Part model, mm, in its own coordinate system. Face numbers are marked on the shaded views. A direction names the side the tool comes from. Coordinates: 2 decimals unless noted, no trailing zeros. Order: outer loops, then holes, each group sorted by start corner. A loop starts at its lowest first (then second) coordinate and runs counter-clockwise, first axis right, second up. Notation, with made-up numbers: (0, 55.25) - (43, 55.25) arc R30 cw to (43, 83.25) - close; hole circle Ø1 at (18.5, 1.5). An arc over 180 degrees is marked (long way). Use a Markdown table: item, result. Add a question column.
1) Saw through at A-A on y = 11. List the corners of the cut face in (x, z), then the cut area to 3 significant figures.
2) Saw through at B-B on x = 15. List the corners of the cut face in (y, z), then the cut area to 3 significant figures.
3) Tool access for the marked faces 5, 6 and 7: list every direction of +Z, -Z, +X, -X, +Y, -Y with a clear straight run to the whole face (end or side of a thin tool).
4) Saw through at C-C on z = 17.5. List the corners of the cut face in (x, y), then the cut area to 3 significant figures.
5) Drop flat-ended pins along their axis: P1, Ø6, axis at x = 21, z = -7, coming from the +Y side; P2, Ø3.5, axis at x = 36.5, y = 15.5, coming from the +Z side; P3, Ø1.6, axis at y = 26, z = 26.5, coming from the +X side. Give the stop position or say it passes through.
6) Two-plate mould, pull along X, no slides. Class the marked faces 1, 2, 3 and 4: +X half, -X half, draft (parallel to the pull), parting line (faces both ways), or undercut.
7) Wall check: L1, parallel to X at y = 11.5, z = -5; L2, parallel to Z at x = -40, y = 21.5; L3, parallel to Z at x = -40, y = 25.5. Give the ranges that are in metal, low to high. Write a range as [from, to].
Autodesk Inventor part; units mm, degrees
ref_plane "YZ Plane" through (0, 0, 0) normal (1, 0, 0) x (0, 1, 0)
ref_plane "XZ Plane" through (0, 0, 0) normal (0, 1, 0) x (-1, 0, 0)
ref_plane "XY Plane" through (0, 0, 0) normal (0, 0, 1) x (1, 0, 0)
sketch "Sketch1" plane through (0, 0, 0) normal (0, 1, 0) x (-1, 0, 0)
  line L0 (42.5, 21.5) -> (-42.5, 21.5)
  line L1 (-42.5, 21.5) -> (-42.5, -21.5)
  line L2 (-42.5, -21.5) -> (42.5, -21.5)
  line L3 (42.5, -21.5) -> (42.5, 21.5)
  point P0 (0, 0)
  point P1 (0, -21.5)
  point P2 (42.5, 0)
  dimension "d0" = 43
  dimension "d1" = 85
extrude "Extrusion1" add sketch "Sketch1" along normal blind 4
sketch "Sketch2" plane through (-42.5, 0, 21.5) normal (0, 0, 1) x (1, 0, 0)
  line L0 (0, 25) -> (85, 25)
  line L1 (85, 25) -> (85, 0)
  line L2 (85, 0) -> (0, 0)
  line L3 (0, 0) -> (0, 25)
  point P0 (42.5, 0)
  dimension "d4" = 25
extrude "Extrusion2" add sketch "Sketch2" along normal blind 2
sketch "Sketch3" plane through (42.5, 0, -21.5) normal (0, 0, -1) x (-1, 0, 0)
  line L0 (0, 25) -> (85, 25)
  line L1 (0, 0) -> (85, 0)
  line L2 (0, 25) -> (85, 25)
  line L3 (85, 25) -> (85, 0)
  line L4 (85, 0) -> (0, 0)
  line L5 (0, 0) -> (0, 25)
  point P0 (42.5, 0)
extrude "Extrusion3" add sketch "Sketch3" along normal blind 2
sketch "Sketch4" plane through (-42.5, 25, -21.5) normal (0, 1, 0) x (1, 0, 0)
  line L0 (0, -45) -> (0, 2)
  line L1 (0, 7.62) -> (85, 7.62)
  line L2 (85, 7.62) -> (85, 0)
  line L3 (85, 0) -> (0, 0)
  line L4 (0, 0) -> (0, 7.62)
  point P0 (42.5, -21.5)
  point P1 (85, 3.81)
  point P2 (85, 2)
  dimension "d15" = 7.62
extrude "Extrusion4" add sketch "Sketch4" along normal blind 2
sketch "Sketch5" plane through (-42.5, 25, 21.5) normal (0, 1, 0) x (1, 0, 0)
  line L0 (0, -2) -> (0, 45)
  line L1 (0, 0) -> (85, 0)
  line L2 (85, 0) -> (85, -7.62)
  line L3 (85, -7.62) -> (0, -7.62)
  line L4 (0, -7.62) -> (0, 0)
  line L5 (85, 0) -> (85, -2)
  line L6 (85, 0) -> (0, 0)
  point P0 (42.5, 21.5)
  point P1 (85, -3.81)
  point P2 (85, -1)
  point P3 (42.5, 0)
  dimension "d17" = 7.62
extrude "Extrusion5" add sketch "Sketch5" along normal blind 2
sketch "Sketch6" plane through (42.5, 0, 23.5) normal (1, 0, 0) x (0, 0, -1)
  line L0 (-5.62, 27) -> (2, 27)
  line L1 (47, 0) -> (47, 25)
  line L2 (0, 27) -> (47, 27)
  line L3 (47, 27) -> (47, 0)
  line L4 (47, 0) -> (0, 0)
  line L5 (0, 0) -> (0, 27)
  line L6 (0, 0) -> (0, 25)
  point P0 (23.5, 0)
  point P1 (0, 13.5)
extrude "Extrusion6" add sketch "Sketch6" along normal blind 2
sketch "Sketch7" plane through (-42.5, 0, -23.5) normal (-1, 0, 0) x (0, 0, 1)
  line L0 (-5.62, 27) -> (2, 27)
  line L1 (47, 25) -> (47, 0)
  line L2 (0, 27) -> (47, 27)
  line L3 (47, 27) -> (47, 0)
  line L4 (47, 0) -> (0, 0)
  line L5 (0, 0) -> (0, 27)
  line L6 (0, 0) -> (0, 25)
  point P0 (23.5, 0)
  point P1 (0, 12.5)
extrude "Extrusion7" add sketch "Sketch7" along normal blind 2
sketch "Sketch8" plane through (-42.5, 27, -21.5) normal (0, 1, 0) x (1, 0, 0)
  circle A0 centre (74.2833, 4.064) radius 1.27
  line L0 (0, 0) -> (85, 0)
  circle A1 centre (51.4233, 4.064) radius 1.27
  circle A2 centre (28.5633, 4.064) radius 1.27
  circle A3 centre (5.7033, 4.064) radius 1.27
  line L1 (95.5719, -20.5867) -> (-13.3282, -20.5867)
  circle A4 centre (74.2833, -45.2374) radius 1.27
  circle A5 centre (51.4233, -45.2374) radius 1.27
  circle A6 centre (28.5633, -45.2374) radius 1.27
  circle A7 centre (5.7033, -45.2374) radius 1.27
  point P0 (42.5, -21.5)
  dimension "d23" = 2.54
  dimension "d24" = 4.064
  dimension "d27" = 22.86
  dimension "d34" = 49.3014
extrude "Extrusion8" cut sketch "Sketch8" against normal through all
properties part number "pruebabateria"
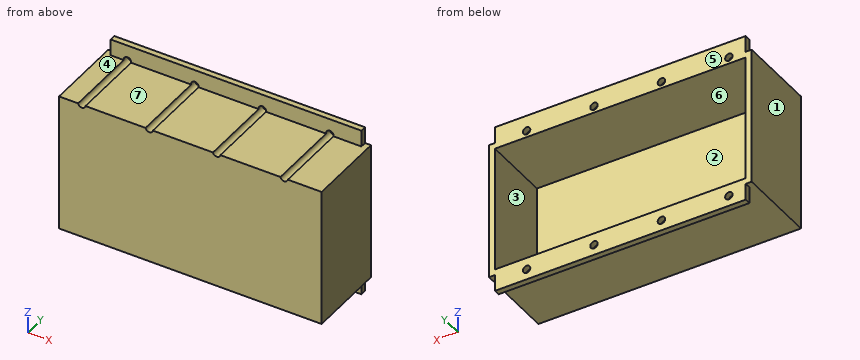
Results are:
| question | item | result |
|---|---|---|
| 1 | outline | (-44.5, -23.5) - (44.5, -23.5) - (44.5, 23.5) - (33.03, 23.5) arc R1.27 cw to (30.54, 23.5) - (10.17, 23.5) arc R1.27 cw to (7.68, 23.5) - (-12.69, 23.5) arc R1.27 cw to (-15.18, 23.5) - (-35.55, 23.5) arc R1.27 cw to (-38.04, 23.5) - (-44.5, 23.5) - close; hole (-42.5, -21.5) - (42.5, -21.5) - (42.5, 21.5) - (-42.5, 21.5) - close |
| 1 | area | 520 mm2 |
| 2 | outline | (0, -23.5) - (25, -23.5) - (25, -29.12) - (27, -29.12) - (27, -21.5) - (4, -21.5) - (4, 21.5) - (27, 21.5) - (27, 29.12) - (25, 29.12) - (25, 23.5) - (0, 23.5) - close |
| 2 | area | 302 mm2 |
| 3 | face 5 | +Z, -Z, +X, -X, +Y |
| 3 | face 6 | +Y |
| 3 | face 7 | +Z, +X, -X, -Y |
| 4 | outline | (-44.5, 0) - (44.5, 0) - (44.5, 27) - (42.5, 27) - (42.5, 4) - (-42.5, 4) - (-42.5, 27) - (-44.5, 27) - close |
| 4 | area | 448 mm2 |
| 5 | P1 | y = 4 |
| 5 | P2 | z = 23.5 |
| 5 | P3 | x = 42.5 |
| 6 | face 1 | -X half |
| 6 | face 2 | undercut |
| 6 | face 3 | undercut |
| 6 | face 4 | draft |
| 7 | L1 | [-44.5, -42.5], [42.5, 44.5] |
| 7 | L2 | [-23.5, -21.5], [21.5, 23.5] |
| 7 | L3 | [-29.12, -21.5], [21.5, 29.12] |
